Input: part model. Units: mm. Frame: model coordinates. A direction names the side the tool comes from. Coordinates: 2 decimals unless noted, no trailing zeros. Loops run counter-clockwise (first coordinate to the right, second up) from the corner with the lowest first, then second, coordinate; pieces in that order, holes last.
Item 1: Section D-D on z = 101. Return loops of the section in (x, y), and give its area (3 significant figures).
Item 2: Ray query, line 1 along Z through (x, y) = (0, -8.25); line 2 along Z through (x, y) = (5, 15.5); line 3 along X through (y, z) = (-13, 100.5). Return the intervals inside material, ascending.
Item 3: Section B-B on y = 3.5. Return loops of the section in (x, z).
Item 4: Section C-C on x = 9. Return loops of the section in (y, z), and give its area (3 significant figures).
Item 5: Reachability of faces 1 (the cylindrical face through (-14.985, 0.66, 65.325)), 2 (the flat face through (0, 0, 117.1)) from +Z, -Z, +X, -X, +Y, -Y: full face, straight path, thin tool, end or side. Return the list, or none.
Item 6: Contact query for flat-ended pins moving along their axis: P1, Ø2, axis at y = -8, z = 56, coming from the -X side; P2, Ø3, axis at x = -12, z = 11.5, coming from the -Y side; P3, Ø8, axis at x = 0, z = 102.1, coming from the +Y side; P4, Ø5.5, axis at x = 0, z = 102.1, coming from the -Y side. Output: stop coordinate, or through.
Item 7: Section A-A on x = 0. Return loops of the section in (y, z).
```python
from build123d import *

# Parameters (mm, degrees)
SKETCH_R          = 22.5
PAD_DEPTH         = 14.98
SKETCH001_R       = 15
PAD001_DEPTH      = 102.12
SKETCH003_R       = 3
POCKET_DEPTH      = 22.501
POCKET_DEPTH_BACK = -22.501


with BuildPart() as part:
    # Sketch → Pad (new body)
    with BuildSketch(Plane.XY):
        Circle(SKETCH_R)
    extrude(amount=PAD_DEPTH)

    # Sketch001 (on Face3 of Pad) → Pad001 (join)
    with BuildSketch(Plane.XY.offset(14.98)):
        Circle(SKETCH001_R)
    extrude(amount=PAD001_DEPTH)

    # Sketch003 → Pocket (cut, two sides)
    with BuildSketch(Plane.XZ) as pocket_sk:
        with Locations((0, 102.1)):
            Circle(SKETCH003_R)
    extrude(amount=-POCKET_DEPTH, mode=Mode.SUBTRACT)
    extrude(pocket_sk.sketch, amount=-POCKET_DEPTH_BACK, mode=Mode.SUBTRACT)


solid = part.part
```
Results found:
1. outline: (-2.79, -14.74) - (-2.79, 14.74) arc R15 ccw to start; (2.79, -14.74) arc R15 ccw to (2.79, 14.74) - close
1. area: 540 mm2
2. line 1: z = 0 to 99.1, 105.1 to 117.1
2. line 2: z = 0 to 14.98
2. line 3: x = -7.48 to -2.54, 2.54 to 7.48
3. outline: (-22.23, 0) - (22.23, 0) - (22.23, 14.98) - (14.59, 14.98) - (14.59, 117.1) - (-14.59, 117.1) - (-14.59, 14.98) - (-22.23, 14.98) - close; hole circle Ø6 at (0, 102.1)
4. outline: (-20.62, 0) - (20.62, 0) - (20.62, 14.98) - (12, 14.98) - (12, 117.1) - (-12, 117.1) - (-12, 14.98) - (-20.62, 14.98) - close
4. area: 3,070 mm2
5. face 1: +Z
5. face 2: +Z, +X, -X, +Y, -Y
6. P1: stops at x = -13.27
6. P2: stops at y = -19.9
6. P3: stops at y = 15
6. P4: passes through
7. outline: (-22.5, 0) - (22.5, 0) - (22.5, 14.98) - (15, 14.98) - (15, 99.1) - (-15, 99.1) - (-15, 14.98) - (-22.5, 14.98) - close; (-15, 105.1) - (15, 105.1) - (15, 117.1) - (-15, 117.1) - close
